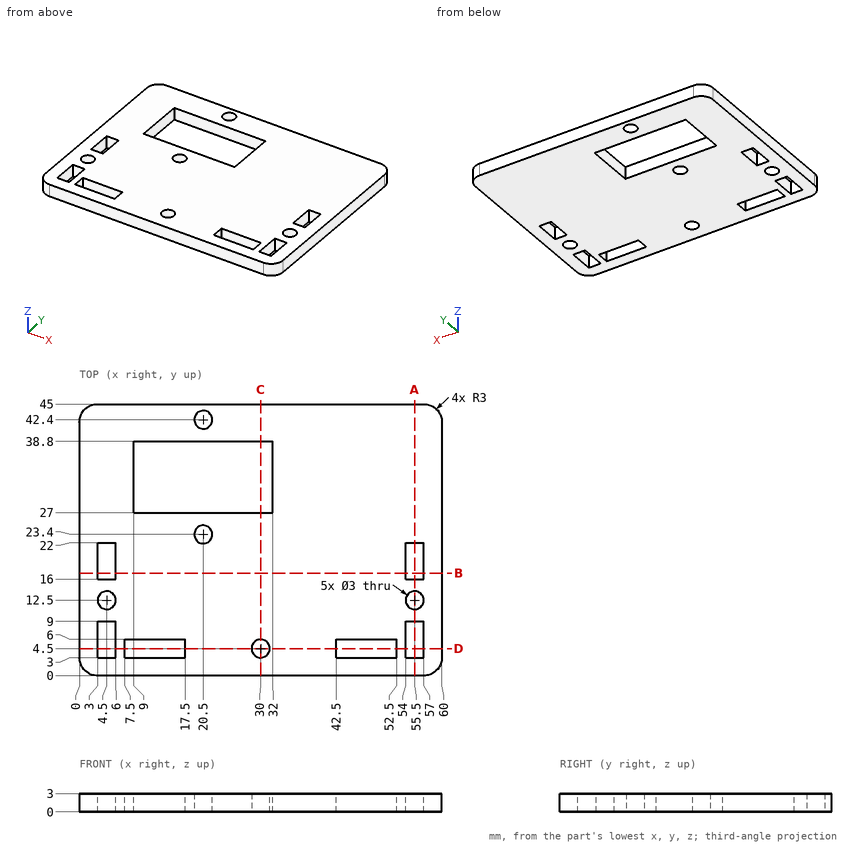
The figure shows three views and two pictorial views of one solid part (mm, origin at its lowest corner). Answer the questions. Coordinates: 2 decimals unless noted, no trailing zeros. Loops run counter-clockwise (first coordinate to the right, second up) from the corner with the lowest first, then second, coordinate; pieces in that order, holes last. Notation, with made-up numbers: (39, 1.5) - (51, 1.5) arc R16 ccw to (51, 31.5) - close; hole circle Ø5 at (14.5, 54). An arc over 180 degrees is marked (long way). Write item = value, one per line.
1) Find the intervals of material crossed by line 1 along Y through (x, z) = (55.5, 0.8); line 2 along X through (y, z) = (8, 0.8); line 3 along Y through (x, z) = (17, 0.55), in increasing order.
Responses:
line_1 = 0 to 3, 9 to 11, 14 to 16, 22 to 45
line_2 = 0 to 3, 6 to 54, 57 to 60
line_3 = 0 to 3, 6 to 27, 38.8 to 45
2) Section A-A (x = 55.5) is taken. Determine the outline of the cut face in (y, z).
Responses:
outline = (0, 0) - (3, 0) - (3, 3) - (0, 3) - close; (9, 0) - (11, 0) - (11, 3) - (9, 3) - close; (14, 0) - (16, 0) - (16, 3) - (14, 3) - close; (22, 0) - (45, 0) - (45, 3) - (22, 3) - close
3) Section D-D (y = 4.5) is taken. Determine the outline of the cut face in (x, z), plus the area to 3 significant figures.
Responses:
outline = (0, 0) - (3, 0) - (3, 3) - (0, 3) - close; (6, 0) - (7.5, 0) - (7.5, 3) - (6, 3) - close; (17.5, 0) - (28.5, 0) - (28.5, 3) - (17.5, 3) - close; (31.5, 0) - (42.5, 0) - (42.5, 3) - (31.5, 3) - close; (52.5, 0) - (54, 0) - (54, 3) - (52.5, 3) - close; (57, 0) - (60, 0) - (60, 3) - (57, 3) - close
area = 93.0 mm^2
4) Section B-B (y = 17) is taken. Determine the outline of the cut face in (x, z).
Responses:
outline = (0, 0) - (3, 0) - (3, 3) - (0, 3) - close; (6, 0) - (54, 0) - (54, 3) - (6, 3) - close; (57, 0) - (60, 0) - (60, 3) - (57, 3) - close
5) Section C-C (x = 30) is taken. Determine the outline of the cut face in (y, z).
Responses:
outline = (0, 0) - (3, 0) - (3, 3) - (0, 3) - close; (6, 0) - (27, 0) - (27, 3) - (6, 3) - close; (38.8, 0) - (45, 0) - (45, 3) - (38.8, 3) - close
